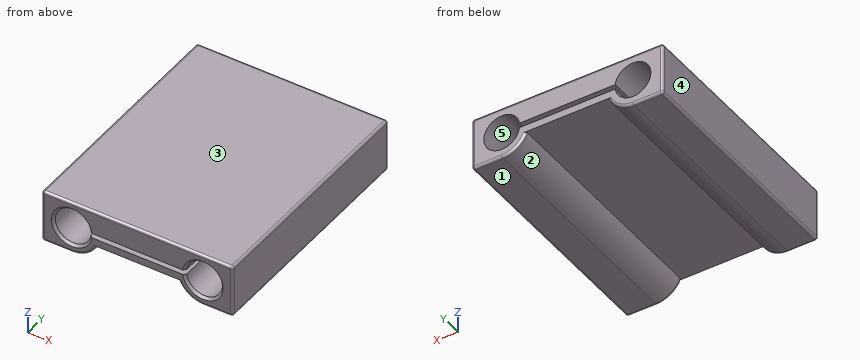
from build123d import *

# Parameters (mm, degrees)
F1_DEPTH = 100
F2_R     = 1
F3_SIZE  = 1


with BuildPart() as f1:
    # F0 (on Front) → F1 (new body)
    with BuildSketch(Plane.XZ):
        with BuildLine():
            Line((39, 11), (-39, 11))
            ThreePointArc((-39, 11), (-39.7071067812, 10.7071067812), (-40, 10))
            Line((-40, 10), (-40, -10))
            ThreePointArc((-40, -10), (-39.7071067812, -10.7071067812), (-39, -11))
            Line((-39, -11), (-27.5, -11))
            ThreePointArc((-27.5, -11), (-21.295163177, -9.0829510623), (-17.253049234, -4))
            Line((-17.253049234, -4), (17.253049234, -4))
            ThreePointArc((17.253049234, -4), (21.295163177, -9.0829510623), (27.5, -11))
            Line((27.5, -11), (39, -11))
            ThreePointArc((39, -11), (39.7071067812, -10.7071067812), (40, -10))
            Line((40, -10), (40, 10))
            ThreePointArc((40, 10), (39.7071067812, 10.7071067812), (39, 11))
        make_face()
        with BuildLine():
            ThreePointArc((-20.0669656263, -1), (-35, 0), (-20.0669656263, 1))
            Line((-20.0669656263, 1), (20.0669656263, 1))
            ThreePointArc((20.0669656263, 1), (35, 0), (20.0669656263, -1))
            Line((20.0669656263, -1), (-20.0669656263, -1))
        make_face(mode=Mode.SUBTRACT)
    extrude(amount=-F1_DEPTH)

    # F2
    f2_edges = [f1.edges().sort_by_distance(p)[0] for p in [
        (39, 50, 11),
        (-39, 50, 11),
        (0, 0, 11),
        (0, 100, 11),
    ]]
    fillet(f2_edges, radius=F2_R)

    # F3
    f3_edges = [f1.edges().sort_by_distance(p)[0] for p in [
        (-35, 0, 0),
        (35, 0, 0),
    ]]
    chamfer(f3_edges, length=F3_SIZE)


solid = f1.part
CAD build for the part. Positions are in the model's coordinates, mm. Face numbers are marked on the shaded views. A direction names the side the tool comes from. Round coordinates to 2 decimals unless told otherwise and drop trailing zeros. Loops run counter-clockwise (first coordinate to the right, second up) from the corner with the lowest first, then second, coordinate; pieces in that order, holes last. Notation, with made-up numbers: (4.25, 62.25) - (18.25, 62.25) arc R21 cw to (18.25, 85.25) - close; hole circle Ø5 at (28.5, 29). An arc over 180 degrees is marked (long way). Put each result on its own line as item: value.
1. Wall check: line 1 (X direction, y = 39, z = 0); line 2 (Z direction, x = -12, y = 62); line 3 (Z direction, x = 27.5, y = 45.5). Give the ranges that are in metal, low to high.
Geometry check:
line 1: -40 to -35, 35 to 40
line 2: -4 to -1, 1 to 11
line 3: -11 to -7.5, 7.5 to 11
2. Pin check, flat tip, straight feed: P1, Ø20, axis at x = 1, y = 72, coming from the -Z side. Stop position of the tip, or through.
Geometry check:
P1: z = -4
3. 3-axis set-ups, long thin cutter, end or side, ignore diameter. For the marked faces 1 and 2: which of +Z, -Z, +X, -X, +Y, -Y reach the whole face in a straight line?
Geometry check:
face 1: -Z, +X, -X, +Y, -Y
face 2: -Z, +Y, -Y
4. Slice it at C-C on z = -2.25. Give the number of separate pieces and of enclosed holes in the cut face, and give its area (3 significant figures).
Geometry check:
separate pieces: 3
enclosed holes: 0
area: 5,140 mm²
5. Two-plate mould, pull along X, no slides. Class the marked faces 3, 4 and 5: released by +X, released by -X, zero draft, split by the parting line, or undercut.
Geometry check:
face 3: zero draft
face 4: released by -X
face 5: undercut
6. Slice it at B-B on y = 86. List the corners of the cut face in (x, z).
Geometry check:
outline: (-40, -10) arc R1 ccw to (-39, -11) - (-27.5, -11) arc R11 ccw to (-17.25, -4) - (17.25, -4) arc R11 ccw to (27.5, -11) - (39, -11) arc R1 ccw to (40, -10) - (40, 10) arc R1 ccw to (39, 11) - (-39, 11) arc R1 ccw to (-40, 10) - close; hole (-20.07, -1) - (20.07, -1) arc R7.5 ccw (long way) to (20.07, 1) - (-20.07, 1) arc R7.5 ccw (long way) to start
7. Slice it at A-A on x = -2. List the corners of the cut face in (y, z).
Geometry check:
outline: (0, -4) - (100, -4) - (100, -1) - (0, -1) - close; (0, 1) - (100, 1) - (100, 10) arc R1 ccw to (99, 11) - (1, 11) arc R1 ccw to (0, 10) - close
